from build123d import *

# Parameters (mm, degrees)
F1_DEPTH = 5.5626
F2_R     = 3.175
F3_DEPTH = 6.08933


with BuildPart() as f1:
    # F0 (on Top) → F1 (new body)
    with BuildSketch(Plane.XY):
        Polygon((-3.207902, -5.55625), (3.207902, -5.55625), (6.415805, 0), (3.207902, 5.55625), (-3.207902, 5.55625), (-6.415805, 0), align=None)
    extrude(amount=F1_DEPTH)

    # F2 (on face) → F3 (cut)
    with BuildSketch(Plane.XY.offset(5.5626)):
        Circle(F2_R)
    extrude(amount=-F3_DEPTH, mode=Mode.SUBTRACT)


solid = f1.part
Geometry check sheet. Reference: the model listing, model coordinates, mm. Round coordinates to 2 decimals unless told otherwise and drop trailing zeros. Loops run counter-clockwise (first coordinate to the right, second up) from the corner with the lowest first, then second, coordinate; pieces in that order, holes last. Notation, with made-up numbers: (62.5, -9.5) - (109.5, -9.5) arc R9 ccw to (109.5, 6.5) - close; hole circle Ø10 at (89, 70). An arc over 180 degrees is marked (long way). One line per question, with ' | ' between items. Start each with the question number.
1. Cross-section at B-B on z = 0.5. Record the cut outline in (x, y) (3 decimals).
2. Scan lines: line 1 (Y direction, x = 0, z = 4.1) (3 decimals); line 2 (Y direction, x = 1, z = 2.4); line 3 (X direction, y = 0.5, z = 1). Record each from-to range of solid material in increasing order. Write a range as [from, to].
3. Draft check along Y on faces 1 (the face through (-0.69, -3.1, 2.82)), 2 (the face through (-4.834, -2.739, 2.742)), 3 (the face through (-4.8, 2.8, 2.7)). Enter one of: released by +Y, released by -Y, zero draft, split by the parting line, or undercut.
4. Depth check by flat-ended pin: pin 1 (1 mm diameter, centred on x = 0.5, y = 0.5, fed in from -Z); pin 2 (1.5 mm diameter, centred on x = -4, z = 4, fed in from +Y). Enter the tip coordinate at first touch or a pass-through.
5. Cross-section at D-D on x = -4. Record the cut outline in (y, z), then the cut area to 3 significant figures.
6. Cross-section at A-A on x = 0. Record the cut outline in (y, z) (3 decimals).
7. Cross-section at C-C on y = 1. Record the cut outline in (x, z).
Taken from the geometry:
1) outline: (-6.416, 0) - (-3.208, -5.556) - (3.208, -5.556) - (6.416, 0) - (3.208, 5.556) - (-3.208, 5.556) - close; hole circle Ø6.35 at (0, 0)
2) line 1: [-5.556, -3.175], [3.175, 5.556] | line 2: [-5.56, -3.01], [3.01, 5.56] | line 3: [-6.13, -3.14], [3.14, 6.13]
3) face 1: undercut | face 2: released by -Y | face 3: released by +Y
4) pin 1: through | pin 2: y = 5.48
5) outline: (-4.18, 0) - (4.18, 0) - (4.18, 5.56) - (-4.18, 5.56) - close | area: 46.6 mm²
6) outline: (-5.556, 0) - (-3.175, 0) - (-3.175, 5.563) - (-5.556, 5.563) - close; (3.175, 0) - (5.556, 0) - (5.556, 5.563) - (3.175, 5.563) - close
7) outline: (-5.84, 0) - (-3.01, 0) - (-3.01, 5.56) - (-5.84, 5.56) - close; (3.01, 0) - (5.84, 0) - (5.84, 5.56) - (3.01, 5.56) - close
